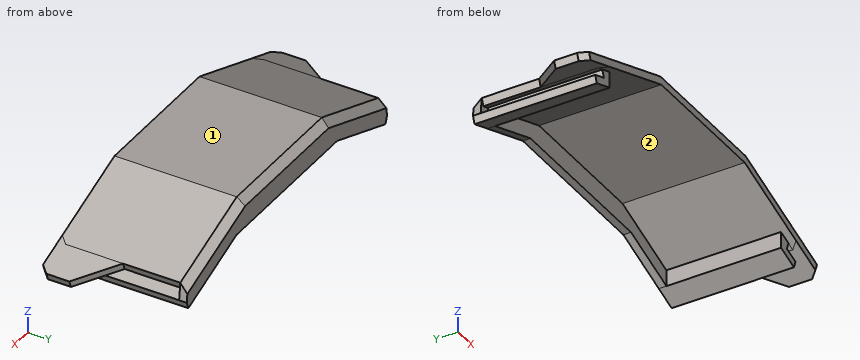
```python
from build123d import *

# Parameters (mm, degrees)
BOSS_EXTRUDE5_DEPTH = 30
BOSS_EXTRUDE6_DEPTH = 2
BOSS_EXTRUDE7_DEPTH = 2
CHAMFER2_SIZE       = 2
CHAMFER3_SIZE       = 2
BOSS_EXTRUDE8_DEPTH = 2
BOSS_EXTRUDE9_DEPTH = 2
CHAMFER4_SIZE       = 2


with BuildPart() as part:
    # Sketch5 → Boss-Extrude5 (new body)
    with BuildSketch(Plane(origin=(0, 0, 0), x_dir=(1, 0, 0), z_dir=(0, 1, 0))):
        Polygon((-40, 10.050874286), (-40.684040287, 8.171489044), (-42.563425528, 8.855529331), (-43.247465815, 6.976144089), (-18.585712616, -2), (18.585712616, -2), (43.247465815, 6.976144089), (42.563425528, 8.855529331), (40.684040287, 8.171489044), (40, 10.050874286), (43.758770483, 11.418954859), (43.074730196, 13.2983401), (37.436574472, 11.24621924), (37.436574472, 6.989508151), (18.233058655, 0), (-18.233058655, 0), (-37.436574472, 6.989508151), (-37.436574472, 11.24621924), (-43.074730196, 13.2983401), (-43.758770483, 11.418954859), align=None)
    extrude(amount=BOSS_EXTRUDE5_DEPTH)

    # Sketch6 → Boss-Extrude6 (add)
    with BuildSketch(Plane(origin=(0, 30, 0), x_dir=(1, 0, 0), z_dir=(0, 1, 0))):
        Polygon((-43.758770483, 11.418954859), (-43.247465815, 6.976144089), (-18.585712616, -2), (18.585712616, -2), (43.247465815, 6.976144089), (43.758770483, 11.418954859), (43.074730196, 13.2983401), (37.436574472, 11.24621924), (21.987207763, 5.62310962), (-21.987207763, 5.62310962), (-37.436574472, 11.24621924), (-43.074730196, 13.2983401), align=None)
    extrude(amount=BOSS_EXTRUDE6_DEPTH)

    # Sketch7 → Boss-Extrude7 (add)
    with BuildSketch(Plane.XZ):
        Polygon((-43.247465815, -6.976144089), (-42.563425528, -8.855529331), (-18.233058655, 0), (18.233058655, 0), (42.563425528, -8.855529331), (43.247465815, -6.976144089), (18.585712616, 2), (-18.585712616, 2), align=None)
    extrude(amount=BOSS_EXTRUDE7_DEPTH)

    # Chamfer2
    chamfer2_edges = [part.edges().sort_by_distance(p)[0] for p in [
        (30.916589216, 32, -2.488072045),
        (0, 32, 2),
        (-30.916589216, 32, -2.488072045),
    ]]
    chamfer(chamfer2_edges, length=CHAMFER2_SIZE)

    # Chamfer3
    chamfer3_edges = [part.edges().sort_by_distance(p)[0] for p in [
        (-42.905445672, -2, -7.91583671),
        (42.905445672, -2, -7.91583671),
    ]]
    chamfer(chamfer3_edges, length=CHAMFER3_SIZE)

    # Sketch10 → Boss-Extrude8 (add)
    with BuildSketch(Plane(origin=(-2.816902982, 0, 7.739377337), x_dir=(0.9396926207859265, 0, 0.34202014332561875), z_dir=(-0.34202014332561875, 0, 0.9396926207859265))):
        Polygon((-41.025306295, -2), (-43.025306295, 0), (-43.025306295, 15), (-52.025306295, 6), (-52.025306295, -2), align=None)
    extrude(amount=-BOSS_EXTRUDE8_DEPTH)

    # Sketch11 → Boss-Extrude9 (add)
    with BuildSketch(Plane(origin=(2.816902982, 0, 7.739377337), x_dir=(0.9396926207859748, 0, -0.342020143325486), z_dir=(0.3420201433254861, 0, 0.9396926207859749))):
        Polygon((41.025306295, -2), (43.025306295, 0), (43.025306295, 15), (52.025306295, 6), (52.025306295, -2), align=None)
    extrude(amount=-BOSS_EXTRUDE9_DEPTH)

    # Chamfer4
    chamfer4_edges = [part.edges().sort_by_distance(p)[0] for p in [
        (-51.362679259, -2, -10.994018),
        (51.362679259, -2, -10.994018),
    ]]
    chamfer(chamfer4_edges, length=CHAMFER4_SIZE)


solid = part.part
```
Geometry: final body of the model. Coordinates: model frame, mm. Face numbers are marked on the shaded views. Round coordinates to 2 decimals unless told otherwise and drop trailing zeros. Order: outer loops, then holes, each group sorted by start corner. A loop starts at its lowest first (then second) coordinate and runs counter-clockwise, first axis right, second up. Notation, with made-up numbers: (-10, 49.25) -> (43, 49.25) arc R30 ccw to (43, 81.25) -> close; hole circle Ø4 at (-8.75, 52). An arc over 180 degrees is marked (long way). Use one line per item in the form item = value. Start each with the question number.
1. Line query: probe 1 along Z at (x, y) = (10.5, 8); probe 2 along Y at (x, z) = (37.5, -8.75); probe 3 along Y at (x, z) = (-27.5, -4.75). Output: solid intervals per line, ascending.
2. Draft query along X for the marked faces 1 and 2. Return one class per face: pulls with the +X half, pulls with the -X half, needs draft (parallel to the pull), parting line crosses it, or undercut.
3. Cut plane C-C (x = 12). Return the cut outline in (y, z).
4. Pin query (flat end, axial travel): pin 1 Ø6 at (x, z) = (13, -4.5) entering from -Y; pin 2 Ø3.5 at (y, z) = (17.5, -8.5) entering from +X; pin 3 Ø2 at (x, y) = (-25, 19) entering from -Z. Return the tip coordinate at first contact, or that it passes through.
5. Cut plane B-B (z = -1). Return the cut outline in (x, y), then the cut area to 3 significant figures.
6. Cut plane A-A (y = 1). Return the cut outline in (x, z), then the cut area to 3 significant figures.
7. Cut plane D-D (y = 17.5). Return the cut outline in (x, z), then the cut area to 3 significant figures.
Solution:
q1.probe_1 = 0 to 2
q1.probe_2 = 0 to 32
q1.probe_3 = 30 to 32
q2.face_1 = needs draft
q2.face_2 = undercut
q3.outline = (-2, 0) -> (30, 0) -> (30, -5.62) -> (32, -5.62) -> (32, 0) -> (30, 2) -> (-2, 2) -> close
q4.pin_1 = 30
q4.pin_2 = 43.25
q4.pin_3 = -2.83
q5.outline = (-26.83, -2) -> (-20.98, -2) -> (-20.98, 30) -> (20.98, 30) -> (20.98, -2) -> (26.83, -2) -> (26.83, 30) -> (20.98, 32) -> (-20.98, 32) -> (-26.83, 30) -> close
q5.area = 470 mm^2
q6.outline = (-51.7, -10.05) -> (-51.02, -11.93) -> (-40.68, -8.17) -> (-40, -10.05) -> (-43.76, -11.42) -> (-43.07, -13.3) -> (-37.44, -11.25) -> (-37.44, -6.99) -> (-18.23, 0) -> (18.23, 0) -> (37.44, -6.99) -> (37.44, -11.25) -> (43.07, -13.3) -> (43.76, -11.42) -> (40, -10.05) -> (40.68, -8.17) -> (51.02, -11.93) -> (51.7, -10.05) -> (18.59, 2) -> (-18.59, 2) -> close
q6.area = 252 mm^2
q7.outline = (-43.76, -11.42) -> (-43.07, -13.3) -> (-37.44, -11.25) -> (-37.44, -6.99) -> (-18.23, 0) -> (18.23, 0) -> (37.44, -6.99) -> (37.44, -11.25) -> (43.07, -13.3) -> (43.76, -11.42) -> (40, -10.05) -> (40.68, -8.17) -> (42.56, -8.86) -> (43.25, -6.98) -> (18.59, 2) -> (-18.59, 2) -> (-43.25, -6.98) -> (-42.56, -8.86) -> (-40.68, -8.17) -> (-40, -10.05) -> close
q7.area = 216 mm^2
